Here's how the part is built. I have some questions about the finished solid (model axes, mm). Give positions to 0.01 mm unless a question says otherwise; leave off trailing zeros. Loops run counter-clockwise (first coordinate to the right, second up) from the corner with the lowest first, then second, coordinate; pieces in that order, holes last. Notation, with made-up numbers: (49, -9.75) - (81, -9.75) arc R21 ccw to (81, 19.25) - close; hole circle Ø11 at (22.25, 3). An arc over 180 degrees is marked (long way). Use one line per item in the form item = value.
from build123d import *

# Parameters (mm, degrees)
F0_R     = 10
F1_DEPTH = 25
F2_DEPTH = 50
F3_SIZE  = 2


with BuildPart() as f1:
    # F0 (on Front) → F1 (new body)
    with BuildSketch(Plane.XZ):
        with BuildLine():
            ThreePointArc((5.994869, -24.27059), (19.683391, -15.413116), (25, 0))
            ThreePointArc((25, 0), (18.399502, 16.92508), (2.083333, 24.913043))
            ThreePointArc((2.083333, 24.913043), (-24.921312, -1.981973), (5.994869, -24.27059))
        make_face()
        Circle(F0_R, mode=Mode.SUBTRACT)
        with BuildLine():
            ThreePointArc((2.083333, 24.913043), (18.399502, 16.92508), (25, 0))
            ThreePointArc((25, 0), (19.683391, -15.413116), (5.994869, -24.27059))
            Line((5.994869, -24.27059), (40.323092, -21.526636))
            Line((40.323092, -21.526636), (91.394378, -17.44436))
            ThreePointArc((91.394378, -17.44436), (72.500029, 0.032084), (91.458333, 17.43913))
            Line((91.458333, 17.43913), (2.083333, 24.913043))
        make_face()
        with BuildLine():
            ThreePointArc((107.5, 0), (102.879651, 11.847556), (91.458333, 17.43913))
            ThreePointArc((91.458333, 17.43913), (72.500029, 0.032084), (91.394378, -17.44436))
            ThreePointArc((91.394378, -17.44436), (102.857908, -11.87115), (107.5, 0))
        make_face()
        with Locations((90, 0)):
            Circle(F0_R, mode=Mode.SUBTRACT)
    extrude(amount=F1_DEPTH)

    # F0 (on Front) → F2 (join)
    with BuildSketch(Plane.XZ):
        with BuildLine():
            ThreePointArc((5.994869, -24.27059), (19.683391, -15.413116), (25, 0))
            ThreePointArc((25, 0), (18.399502, 16.92508), (2.083333, 24.913043))
            ThreePointArc((2.083333, 24.913043), (-24.921312, -1.981973), (5.994869, -24.27059))
        make_face()
        Circle(F0_R, mode=Mode.SUBTRACT)
    extrude(amount=F2_DEPTH)

    # F3
    f3_edges = [f1.edges().sort_by_distance(p)[0] for p in [
        (-5.994869, -50, 24.27059),
        (-10, -50, 0),
        (80, -25, 0),
    ]]
    chamfer(f3_edges, length=F3_SIZE)


solid = f1.part
(1) Thinking about a two-plate mould opening in Z: for faces 1 (the flat face through (47.396, -12.325, 21.124)), 2 (the flat face through (10, -50, -10)), 3 (the conical face through (-2.195, -48.125, -9.884)), which applies, pulls with the +Z half, pulls with the -Z half, needs draft (parallel to the pull), parting line crosses it, or undercut?
Geometry says:
face_1 = pulls with the +Z half
face_2 = needs draft
face_3 = undercut
(2) If we section it at D-D (x = 45): List the corners of the cut face in (y, z) for me, plus the area to 3 significant figures.
Geometry says:
outline = (-25, -21.15) - (0, -21.15) - (0, 21.32) - (-25, 21.32) - close
area = 1,060 mm²
(3) For P1, Ø18, axis at x = 0, z = 0, coming from the +Y side; P2, Ø1.5, axis at x = 54.5, y = -23.5, coming from the -Z side; P3, Ø2, axis at x = 4.5, y = -17, coming from the +Z side; P4, Ø2, axis at y = -15, z = -13, coming from the +X side, each with a flat end and sliding along its axis, tell me the tip position at first contact or that it passes through.
Geometry says:
P1 = through
P2 = -20.45
P3 = 24.79
P4 = 102.74
(4) If we section it at B-B (x = 90): List the corners of the cut face in (y, z) for me, plus the area to 3 significant figures.
Geometry says:
outline = (-25, -17.56) - (0, -17.56) - (0, -10) - (-23, -10) - (-25, -12) - close; (-25, 12) - (-23, 10) - (0, 10) - (0, 17.56) - (-25, 17.56) - close
area = 374 mm²
(5) If I drill on probe 1 along Z at (x, y) = (0, -18.5); probe 2 along Y at (x, z) = (55.5, -14); probe 3 along Z at (x, y) = (90, -16), over which ranges is the centre line in solid material (lowest first)?
Geometry says:
probe_1 = -25 to -10, 10 to 25
probe_2 = -25 to 0
probe_3 = -17.56 to -10, 10 to 17.56
(6) If we section it at C-C (z = -2.5): Give the number of separate pieces and of enclosed holes in the cut face, plus the area to 3 significant figures.
Geometry says:
separate_pieces = 3
enclosed_holes = 0
area = 3,080 mm²
(7) If we section it at A-A (y = -4.5): List the corners of the cut face in (x, z) for me, plus the area to 3 significant figures.
Geometry says:
outline = (2.08, 24.91) arc R25 ccw (long way) to (5.99, -24.27) - (91.39, -17.44) arc R17.5 ccw to (91.46, 17.44) - close; hole circle Ø20 at (0, 0); hole circle Ø20 at (90, 0)
area = 4,660 mm²
